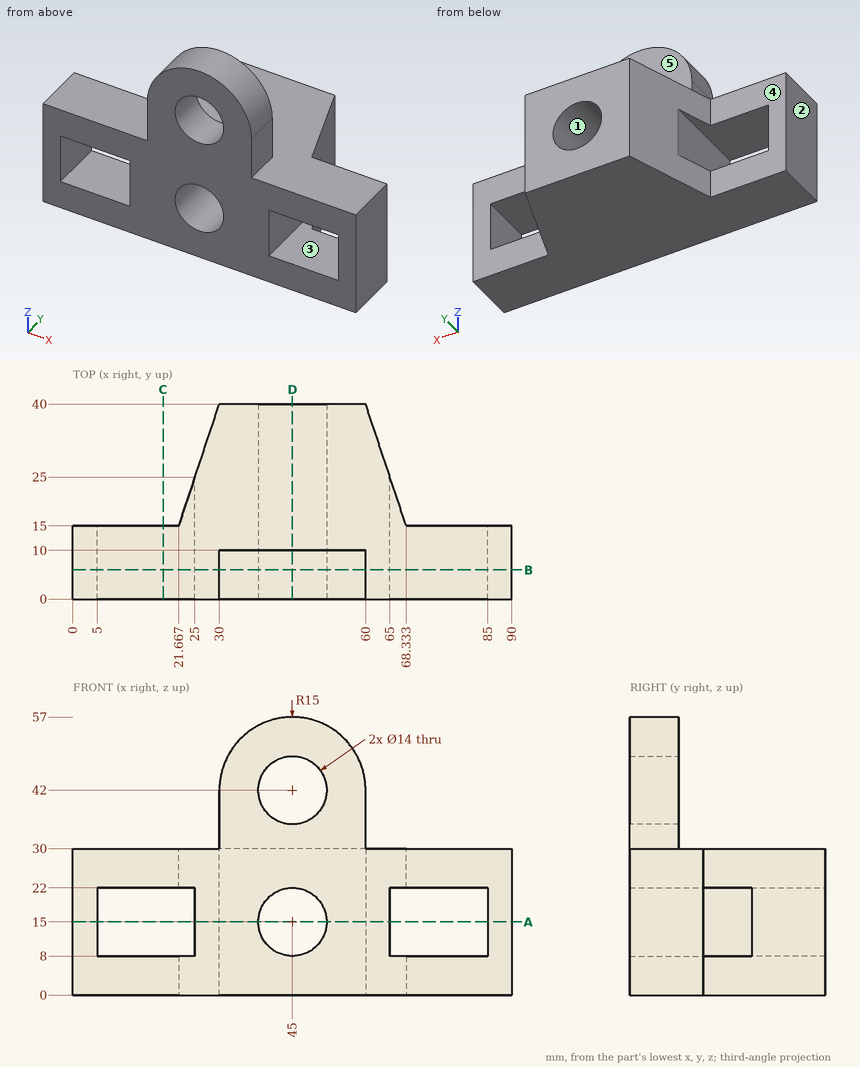
For this review, use the dimensioned drawing (mm, ordinates from the lowest corner) and the shaded views. A direction names the side the tool comes from. Give positions to 0.01 mm unless a question says otherwise; leave off trailing zeros. Write each loop counter-clockwise with the first axis right and the second up, starting at its lowest first coordinate (ties: lowest second). Pieces come first, ordered by that corner, then holes.
(1) To check wall thickness, follow L1, parallel to X at y = 6, z = 42; L2, parallel to Z at x = 41, y = 6.5 (1 decimal); L3, parallel to X at y = 22, z = 15. State the ranges of each line that lie inside material, in increasing order.
(2) The part is to be moulded in two halves that separate along Z. For the marked faces 1 and 2, say which applies: released by +Z, released by -Z, zero draft, split by the parting line, or undercut.
(3) Consider section C-C, the plane x = 18.5. Give the boundary of the cut face in (y, z).
(4) Consider section B-B, the plane y = 6. Give the boundary of the cut face in (x, z).
(5) Consider section D-D, the plane x = 45. Give the boundary of the cut face in (y, z), and give its area (3 significant figures).
(6) For P1, Ø24, axis at x = 8.5, z = 17.5, coming from the +Y side; P2, Ø3, axis at x = 56, y = 5, coming from the +Z side; P3, Ø22, axis at x = 74.5, y = 17.5, coming from the +Z side, all flat-tipped, find the tip position at first contact; note any pin that passes through.
(7) Consider section A-A, the plane z = 15. Give the boundary of the cut face in (x, y), and give its area (4 significant figures).
(8) Tool access review of the marked faces 3, 4 and 5: name each direction out of +Z, -Z, +X, -X, +Y, -Y from which nothing blocks a thin tool from reaching the whole face with its end or side.
Returned:
1. L1: x = 30 to 38, 52 to 60
1. L2: z = 0 to 9.3, 20.7 to 36.3, 47.7 to 56.5
1. L3: x = 25 to 38, 52 to 65
2. face 1: undercut
2. face 2: zero draft
3. outline: (0, 0) - (15, 0) - (15, 8) - (0, 8) - close; (0, 22) - (15, 22) - (15, 30) - (0, 30) - close
4. outline: (0, 0) - (90, 0) - (90, 30) - (60, 30) - (60, 42) arc R15 ccw to (30, 42) - (30, 30) - (0, 30) - close; hole (5, 8) - (25, 8) - (25, 22) - (5, 22) - close; hole circle Ø14 at (45, 15); hole circle Ø14 at (45, 42); hole (65, 8) - (85, 8) - (85, 22) - (65, 22) - close
5. outline: (0, 0) - (40, 0) - (40, 8) - (0, 8) - close; (0, 22) - (40, 22) - (40, 30) - (10, 30) - (10, 35) - (0, 35) - close; (0, 49) - (10, 49) - (10, 57) - (0, 57) - close
5. area: 770 mm2
6. P1: stops at y = 15
6. P2: stops at z = 53.61
6. P3: stops at z = 30
7. outline: (0, 0) - (5, 0) - (5, 15) - (0, 15) - close; (25, 0) - (38, 0) - (38, 40) - (30, 40) - (25, 25) - close; (52, 0) - (65, 0) - (65, 25) - (60, 40) - (52, 40) - close; (85, 0) - (90, 0) - (90, 15) - (85, 15) - close
7. area: 1,115 mm2
8. face 3: +Y, -Y
8. face 4: +Z, -Z, -X, +Y
8. face 5: +Z, +X, -X, +Y
